Geometry check sheet. Reference: drawing and pictorial views, mm from the part's lowest x, y, z. A direction names the side the tool comes from. Give positions to 0.01 mm unless a question says otherwise; leave off trailing zeros. Loops run counter-clockwise (first coordinate to the right, second up) from the corner with the lowest first, then second, coordinate; pieces in that order, holes last. Notation, with made-up numbers: M 63,-34.75 L 109,-34.75 A23 cw 109,-13.75 Z; hole C 77,-15 d8. An arc over 180 degrees is marked long. Use CSV: the item, a comma, the result in double quotes.
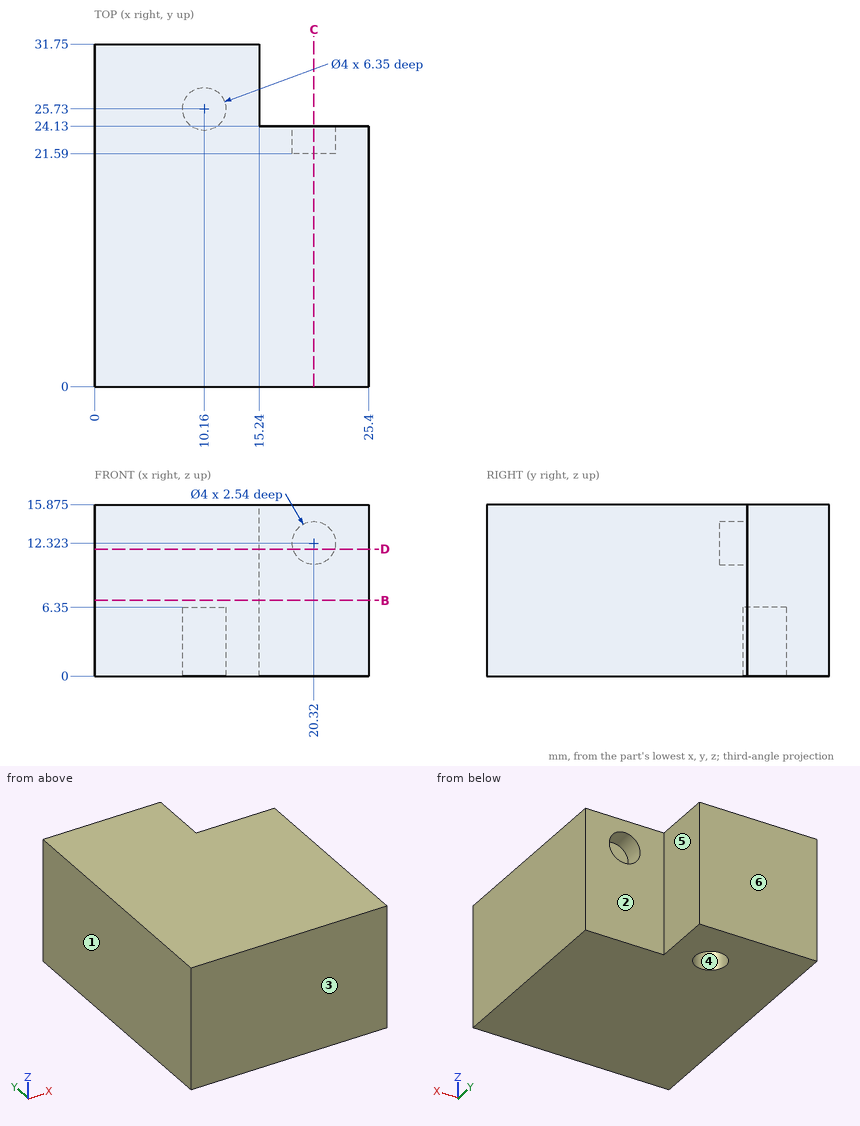
(1) Section check C-C on x = 20.32. Record the cut outline in (y, z) (1 decimal), plus the area to 3 significant figures.
Calculated:
outline,"M 0,0 L 24.1,0 L 24.1,10.3 L 21.6,10.3 L 21.6,14.3 L 24.1,14.3 L 24.1,15.9 L 0,15.9 Z"
area,"373 mm²"
(2) Scan lines: L1, parallel to Y at x = 10.16, z = 4.5; L2, parallel to Z at x = 20.32, y = 22.6 (1 decimal); L3, parallel to Y at x = 19.75, z = 7. Record each from-to range of solid material in increasing order. Write a range as from..to.
Calculated:
L1,"y = 0..23.73, 27.73..31.75"
L2,"z = 0..10.3, 14.3..15.9"
L3,"y = 0..24.13"
(3) Section check D-D on z = 11.75. Record the cut outline in (x, y).
Calculated:
outline,"M 0,0 L 25.4,0 L 25.4,24.13 L 22.24,24.13 L 22.24,21.59 L 18.4,21.59 L 18.4,24.13 L 15.24,24.13 L 15.24,31.75 L 0,31.75 Z"
(4) Section check B-B on z = 7. Record the cut outline in (x, y), plus the area to 3 significant figures.
Calculated:
outline,"M 0,0 L 25.4,0 L 25.4,24.13 L 15.24,24.13 L 15.24,31.75 L 0,31.75 Z"
area,"729 mm²"
(5) Tool access check on the marked faces 1 and 2. Record the directions out of +Z, -Z, +X, -X, +Y, -Y that give a thin tool (end or side, any length) a straight path to the whole face; none if there is none.
Calculated:
face 1,"+Z, -Z, -X, +Y, -Y"
face 2,"+Z, -Z, +X, +Y"
(6) Mould release check, pull along Y, two halves, no side actions. Record for the marked faces 3, 4, 5 and 6: released by +Y, released by -Y, zero draft, split by the parting line, or undercut.
Calculated:
face 3,"released by -Y"
face 4,"undercut"
face 5,"zero draft"
face 6,"released by +Y"
(7) Depth check by flat-ended pin: pin 1 Ø2.5 at (y, z) = (28.5, 6.5) entering from +X; pin 2 Ø4.5 at (x, y) = (10.5, 25) entering from -Z; pin 3 Ø3 at (x, y) = (10.16, 25.73) entering from -Z; pin 4 Ø1.2 at (x, z) = (21.5, 12) entering from +Y. Enter the tip coordinate at first touch or a pass-through.
Calculated:
pin 1,"stops at x = 15.24"
pin 2,"stops at z = 0"
pin 3,"stops at z = 6.35"
pin 4,"stops at y = 21.59"
